Autodesk Inventor part; units mm, degrees
ref_plane "YZ Plane" through (0, 0, 0) normal (1, 0, 0) x (0, 1, 0)
ref_plane "XZ Plane" through (0, 0, 0) normal (0, 1, 0) x (-1, 0, 0)
ref_plane "XY Plane" through (0, 0, 0) normal (0, 0, 1) x (1, 0, 0)
sketch "Sketch1" plane through (0, 0, 0) normal (0, 0, 1) x (1, 0, 0)
  circle A0 centre (10, 24.7) radius 1.6
  line L0 (0, 0) -> (20.0001, 0)
  line L1 (0, 0) -> (0, 7)
  line L2 (20.0001, 0) -> (20.0001, 6.9998)
  line L3 (0, 7) -> (4.9176, 25.3526)
  line L4 (0, 7) -> (19, 7) construction
  line L5 (20.0001, 6.9998) -> (15.0825, 25.3524)
  line L6 (20.0001, 6.9998) -> (39.0001, 6.9998) construction
  arc A1 (15.0825, 25.3524) -> (4.9176, 25.3526) centre (10, 23.9906) ccw
  dimension "d17" = 7
  dimension "d18" = 6.9998
  dimension "d19" = 24.7
  dimension "d23" = 90
  dimension "d24" = 90
  dimension "d25" = 10
  dimension "d26" = 19
  dimension "d27" = 75
  dimension "d28" = 19
  dimension "d29" = 105
  dimension "d30" = 10
sketch "Sketch3" plane through (0, 0, 0) normal (0, 0, 1) x (1, 0, 0)
  point P0 (0, 0)
extrude "Extrusion1" add sketch "Sketch1" along normal blind 4.5
sketch "Sketch4" plane through (0, 0, 4.5) normal (0, 0, 1) x (1, 0, 0)
  line L0 (0, 7) -> (0, 0)
  line L1 (20.0001, 0) -> (20.0001, 6.9998)
  line L2 (0, 0) -> (20.0001, 0)
  line L3 (20.0001, 0) -> (20.0001, 6.9998)
  line L4 (3.884, 22.9404) -> (-0.0481, 7.0119)
  line L5 (20.0001, 6.9998) -> (0, 6.9998)
  line L6 (0, 7) -> (0, 0)
extrude "Extrusion2" add sketch "Sketch4" along normal blind 4.5
sketch "Sketch5" plane through (0, 0, 0) normal (0, -1, 0) x (1, 0, 0)
  circle A0 centre (5, 4) radius 0.5
  circle A1 centre (15, 4) radius 0.5
  line L0 (0, 0) -> (20.0001, 0)
  line L1 (0, 9) -> (20.0001, 9)
  dimension "d13" = 1
  dimension "d14" = 1
  dimension "d33" = 5
  dimension "d34" = 5
extrude "Extrusion3" cut sketch "Sketch5" against normal blind 5.5
properties part number "upper_deck_shaft_mount_for_AD"
Design review of the part built by this model. Coordinates are the model's own, in mm. A direction names the side the tool comes from. Coordinates: 2 decimals unless noted, no trailing zeros. Order: outer loops, then holes, each group sorted by start corner. A loop starts at its lowest first (then second) coordinate and runs counter-clockwise, first axis right, second up. Notation, with made-up numbers: (32.5, -36) -> (76.5, -36) arc R36 cw to (76.5, 3) -> close; hole circle Ø3 at (2.25, 88). An arc over 180 degrees is marked (long way). One line per item, written item: value.
1) We need section B-B, the plane x = 9.5. Give the boundary of the cut face in (y, z).
Output values:
outline: (0, 0) -> (23.18, 0) -> (23.18, 4.5) -> (7, 4.5) -> (7, 9) -> (0, 9) -> close; (26.22, 0) -> (29.23, 0) -> (29.23, 4.5) -> (26.22, 4.5) -> close
2) Clearance check with flat-ended pins moving along their axes: P1, Ø4, axis at x = 10, y = 24.7, coming from the +Z side; P2, Ø0.5, axis at x = 15, z = 4, coming from the -Y side; P3, Ø5, axis at x = 6.5, z = 6.5, coming from the +Y side. State where each tip first meets the part, or that it passes through.
Output values:
P1: stops at z = 4.5
P2: stops at y = 5.5
P3: stops at y = 28.86
3) Draft analysis for pull direction Z (two halves, no side actions). For faces 1 (the face through (10, 16, 4.5)), 2 (the face through (8.4, 24.63, 2.22)), 3 (the face through (15, 5.5, 4)), state which applies: +Z half, -Z half, draft (parallel to the pull), parting line (faces both ways), or undercut.
Output values:
face 1: +Z half
face 2: draft
face 3: undercut
4) We need section C-C, the plane y = 26. Give the boundary of the cut face in (x, z), then the cut area to 3 significant figures.
Output values:
outline: (5.14, 0) -> (9.07, 0) -> (9.07, 4.5) -> (5.14, 4.5) -> close; (10.93, 0) -> (14.86, 0) -> (14.86, 4.5) -> (10.93, 4.5) -> close
area: 35.4 mm2
5) We need section D-D, the plane z = 4. Give the boundary of the cut face in (x, y), then the cut area to 3 significant figures.
Output values:
outline: (0, 0) -> (4.5, 0) -> (4.5, 5.5) -> (5.5, 5.5) -> (5.5, 0) -> (14.5, 0) -> (14.5, 5.5) -> (15.5, 5.5) -> (15.5, 0) -> (20, 0) -> (20, 7) -> (15.08, 25.35) arc R5.26 ccw to (4.92, 25.35) -> (0, 7) -> close; hole circle Ø3.2 at (10, 24.7)
area: 427 mm2
6) We need section A-A, the plane z = 2. Give the boundary of the cut face in (x, y).
Output values:
outline: (0, 0) -> (20, 0) -> (20, 7) -> (15.08, 25.35) arc R5.26 ccw to (4.92, 25.35) -> (0, 7) -> close; hole circle Ø3.2 at (10, 24.7)
7) To check wall thickness, follow probe 1 along Y at (x, z) = (10, 2.2); probe 2 along Z at (x, y) = (5, 4.4); probe 3 along Y at (x, z) = (17.5, 6). State the ranges of each line that lie inside material, in increasing order. Write a range as [from, to].
Output values:
probe 1: y = [0, 23.1], [26.3, 29.25]
probe 2: z = [0, 3.5], [4.5, 9]
probe 3: y = [0, 7]
8) Machinability: for faces 4 (the face through (4.935, 2.712, 4.496)), 5 (the face through (20, 3, 4)), which of the approach directions +Z, -Z, +X, -X, +Y, -Y give a long, thin tool a straight path to every point of the face, cutting with its end or side? Answer none if there is none.
Output values:
face 4: -Y
face 5: +Z, -Z, +X, +Y, -Y
